Could you check a few things on this model? Use its own coordinates, in mm. Round coordinates to 2 decimals unless told otherwise and drop trailing zeros. Loops run counter-clockwise (first coordinate to the right, second up) from the corner with the lowest first, then second, coordinate; pieces in that order, holes last.
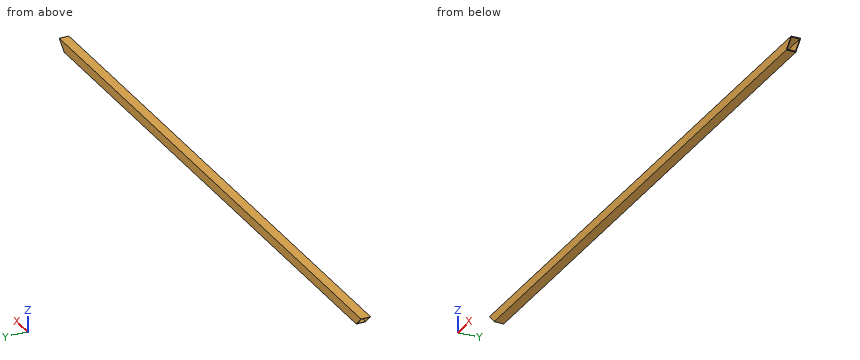
from build123d import *

# Parameters (mm, degrees)
SKETCH1_W           = 25.4
SKETCH1_H           = 25.4
SKETCH1_W_2         = 22.225
SKETCH1_H_2         = 22.225
BOSS_EXTRUDE1_DEPTH = 1574.8
CUT_EXTRUDE1_DEPTH  = 1576.056027575


with BuildPart() as part:
    # Sketch1 → Boss-Extrude1 (new body)
    with BuildSketch(Plane(origin=(0, 0, 0), x_dir=(0, 0, -1), z_dir=(1, 0, 0))):
        Rectangle(SKETCH1_W, SKETCH1_H)
        Rectangle(SKETCH1_W_2, SKETCH1_H_2, mode=Mode.SUBTRACT)
    extrude(amount=BOSS_EXTRUDE1_DEPTH)

    # Sketch2 → Cut-Extrude1 (cut, through all)
    with BuildSketch(Plane(origin=(0, 12.7, 0), x_dir=(1, 0, 0), z_dir=(0, 1, 0))):
        Polygon((0, -12.7), (25.4, 12.7), (0, 12.7), align=None)
    cut_extrude1 = extrude(amount=-CUT_EXTRUDE1_DEPTH, mode=Mode.SUBTRACT)

    # Mirror1: Cut-Extrude1 across plane
    add(cut_extrude1.mirror(Plane(origin=(787.4, 0, 0), x_dir=(0, 0, 1), z_dir=(1, 0, 0))), mode=Mode.SUBTRACT)


solid = part.part
Item 1: If we section it at B-B, the plane x = 723.5: Please give me the cut outline in (y, z).
Results list:
outline: (-12.7, -12.7) - (12.7, -12.7) - (12.7, 12.7) - (-12.7, 12.7) - close; hole (-11.11, -11.11) - (11.11, -11.11) - (11.11, 11.11) - (-11.11, 11.11) - close
Item 2: If I drill on line 1 along Y through (x, z) = (1147, 6.25), over which ranges is the centre line in solid material (lowest first)?
Results list:
line 1: y = -12.7 to -11.11, 11.11 to 12.7
Item 3: If we section it at A-A, the plane z = 0.75: Please give me the cut outline in (x, y), then the cut area to 3 significant figures.
Results list:
outline: (11.95, -12.7) - (1562.85, -12.7) - (1562.85, -11.11) - (11.95, -11.11) - close; (11.95, 11.11) - (1562.85, 11.11) - (1562.85, 12.7) - (11.95, 12.7) - close
area: 4,920 mm2
Item 4: If we section it at C-C, the plane y = 1: Please give me the cut outline in (x, z), then the cut area to 3 significant figures.
Results list:
outline: (0, 12.7) - (1.59, 11.11) - (1573.21, 11.11) - (1574.8, 12.7) - close; (23.81, -11.11) - (25.4, -12.7) - (1549.4, -12.7) - (1550.99, -11.11) - close
area: 4,920 mm2
